Verification items for the finished model (mm, model axes). Face numbers are marked on the shaded views. A direction names the side the tool comes from. Give positions to 0.01 mm unless a question says otherwise; leave off trailing zeros. Write each loop counter-clockwise with the first axis right and the second up, starting at its lowest first coordinate (ties: lowest second). Pieces come first, ordered by that corner, then holes. Notation, with made-up numbers: (83.25, 39) -> (100.25, 39) arc R16 cw to (100.25, 63) -> close; hole circle Ø9 at (-25, 58). An arc over 180 degrees is marked (long way). Write item = value, one per line.
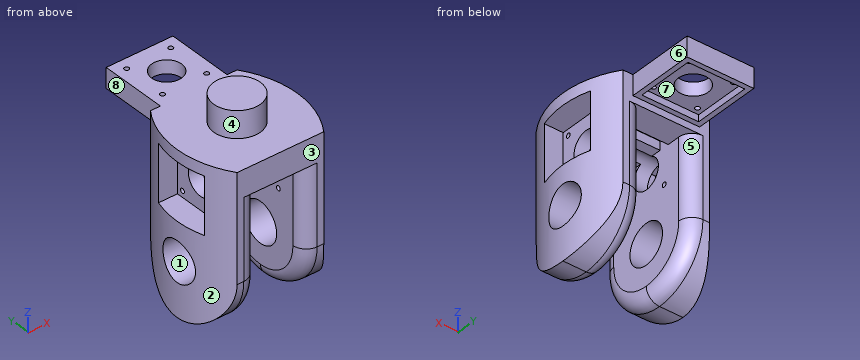
from build123d import *

# Parameters (mm, degrees)
BOSS_EXTRUDE1_DEPTH     = 100
BOSS_EXTRUDE1_2_DEPTH   = 100
BOSS_EXTRUDE2_DEPTH     = 20
SKETCH3_R               = 15
SKETCH3_R_2             = 11.25
SKETCH3_R_3             = 1.75
CUT_EXTRUDE1_DEPTH      = 46
CUT_EXTRUDE1_DEPTH_BACK = 46
SKETCH4_W               = 42.5
SKETCH4_H               = 42.5
CUT_EXTRUDE2_DEPTH      = 17.5
SKETCH5_W               = 42.5
SKETCH5_H               = 42.5
CUT_EXTRUDE4_DEPTH      = 17.5
SKETCH6_W               = 50
SKETCH6_H               = 15
BOSS_EXTRUDE3_DEPTH     = 50
SKETCH7_R               = 11.25
SKETCH7_R_2             = 1.75
CUT_EXTRUDE5_DEPTH      = 106.0000001
CUT_EXTRUDE5_DEPTH_BACK = 16.0000001
SKETCH8_W               = 42.5
SKETCH8_H               = 42.5
CUT_EXTRUDE6_DEPTH      = 5
SKETCH9_R               = 17.5
BOSS_EXTRUDE4_DEPTH     = 20
FILLET1_R               = 10
CUT_EXTRUDE7_DEPTH      = 17.5
CUT_EXTRUDE7_DEPTH_BACK = 17.5


with BuildPart() as part:
    # Sketch1 → Boss-Extrude1 (new body)
    with BuildSketch(Plane.XY):
        with BuildLine():
            Line((-17.5, -40), (-17.5, 40))
            Line((-17.5, 40), (-32.5, 40))
            ThreePointArc((-32.5, 40), (-45, 0), (-32.5, -40))
            Line((-32.5, -40), (-17.5, -40))
        make_face()
    extrude(amount=BOSS_EXTRUDE1_DEPTH)



with BuildPart() as body_2:
    # Sketch1 → Boss-Extrude1 2 (new body)
    with BuildSketch(Plane.XY):
        with BuildLine():
            Line((17.5, -40), (17.5, 40))
            Line((17.5, 40), (32.5, 40))
            ThreePointArc((32.5, 40), (45, 0), (32.5, -40))
            Line((32.5, -40), (17.5, -40))
        make_face()
    extrude(amount=BOSS_EXTRUDE1_2_DEPTH)


with BuildPart() as part_1:
    add(part.part)

    add(body_2.part)  # Boss-Extrude2 merges body 2
    # Sketch2 → Boss-Extrude2 (add)
    with BuildSketch(Plane.XY.offset(100)):
        with BuildLine():
            Line((-32.5, 40), (32.5, 40))
            ThreePointArc((32.5, 40), (45, 0), (32.5, -40))
            Line((32.5, -40), (-32.5, -40))
            ThreePointArc((-32.5, -40), (-45, 0), (-32.5, 40))
        make_face()
    extrude(amount=BOSS_EXTRUDE2_DEPTH)

    # Sketch3 → Cut-Extrude1 (cut, two sides)
    with BuildSketch(Plane(origin=(0, 0, 0), x_dir=(0, 0, -1), z_dir=(1, 0, 0))) as cut_extrude1_sk:
        with BuildLine():
            ThreePointArc((-40, 40), (-11.715728753, 28.284271247), (0, 0))
            Line((0, 0), (0, 40))
            Line((0, 40), (-40, 40))
        make_face()
        with BuildLine():
            Line((0, -40), (0, 0))
            ThreePointArc((0, 0), (-11.715728753, -28.284271247), (-40, -40))
            Line((-40, -40), (0, -40))
        make_face()
        with Locations((-40, 0)):
            Circle(SKETCH3_R)
        with Locations((-90, 0)):
            Circle(SKETCH3_R_2)
        with Locations((-73.45, -16.55)):
            Circle(SKETCH3_R_3)
        with Locations((-73.45, 16.55)):
            Circle(SKETCH3_R_3)
        with Locations((-106.55, 16.55)):
            Circle(SKETCH3_R_3)
        with Locations((-106.55, -16.55)):
            Circle(SKETCH3_R_3)
    extrude(amount=CUT_EXTRUDE1_DEPTH, mode=Mode.SUBTRACT)
    extrude(cut_extrude1_sk.sketch, amount=-CUT_EXTRUDE1_DEPTH_BACK, mode=Mode.SUBTRACT)

    # Sketch4 → Cut-Extrude2 (cut)
    with BuildSketch(Plane(origin=(45, 0, 0), x_dir=(0, 0, -1), z_dir=(1, 0, 0))):
        with Locations((-90, 0)):
            Rectangle(SKETCH4_W, SKETCH4_H)
    extrude(amount=-CUT_EXTRUDE2_DEPTH, mode=Mode.SUBTRACT)

    # Sketch5 → Cut-Extrude4 (cut)
    with BuildSketch(Plane(origin=(-45, 0, 0), x_dir=(0, 0, -1), z_dir=(1, 0, 0))):
        with Locations((-90, 0)):
            Rectangle(SKETCH5_W, SKETCH5_H)
    extrude(amount=CUT_EXTRUDE4_DEPTH, mode=Mode.SUBTRACT)

    # Sketch6 → Boss-Extrude3 (add)
    with BuildSketch(Plane(origin=(0, 40, 0), x_dir=(1, 0, 0), z_dir=(0, 1, 0))):
        with Locations((0, -112.5)):
            Rectangle(SKETCH6_W, SKETCH6_H)
    extrude(amount=BOSS_EXTRUDE3_DEPTH)

    # Sketch7 → Cut-Extrude5 (cut, two sides)
    with BuildSketch(Plane(origin=(0, 0, 105), x_dir=(-1, 0, 0), z_dir=(0, 0, -1))) as cut_extrude5_sk:
        with Locations((0, 65)):
            Circle(SKETCH7_R)
        with Locations((16.55, 81.55)):
            Circle(SKETCH7_R_2)
        with Locations((-16.55, 81.55)):
            Circle(SKETCH7_R_2)
        with Locations((-16.55, 48.45)):
            Circle(SKETCH7_R_2)
        with Locations((16.55, 48.45)):
            Circle(SKETCH7_R_2)
    extrude(amount=CUT_EXTRUDE5_DEPTH, mode=Mode.SUBTRACT)
    extrude(cut_extrude5_sk.sketch, amount=-CUT_EXTRUDE5_DEPTH_BACK, mode=Mode.SUBTRACT)

    # Sketch8 → Cut-Extrude6 (cut)
    with BuildSketch(Plane(origin=(0, 0, 105), x_dir=(-1, 0, 0), z_dir=(0, 0, -1))):
        with Locations((0, 65)):
            Rectangle(SKETCH8_W, SKETCH8_H)
    extrude(amount=-CUT_EXTRUDE6_DEPTH, mode=Mode.SUBTRACT)

    # Sketch9 → Boss-Extrude4 (add)
    with BuildSketch(Plane.XY.offset(120)):
        Circle(SKETCH9_R)
    extrude(amount=BOSS_EXTRUDE4_DEPTH)

    # Fillet1
    fillet1_edges = [part_1.edges().sort_by_distance(p)[0] for p in [
        (17.5, 40, 70),
        (17.5, -40, 70),
        (-17.5, 0, 0),
        (17.5, 0, 0),
        (-17.5, 40, 70),
        (-17.5, -40, 70),
    ]]
    fillet(fillet1_edges, radius=FILLET1_R)

    # Sketch10 → Cut-Extrude7 (cut, two sides)
    with BuildSketch(Plane(origin=(0, 0, 0), x_dir=(0, 0, -1), z_dir=(1, 0, 0))) as cut_extrude7_sk:
        with BuildLine():
            Line((-106.55, 20.3), (-92.703309556, 20.3))
            Line((-92.703309556, 20.3), (-92.703309556, 12.8))
            Line((-92.703309556, 12.8), (-106.55, 12.8))
            ThreePointArc((-106.55, 12.8), (-110.3, 16.55), (-106.55, 20.3))
        make_face()
        with BuildLine():
            Line((-106.55, -12.8), (-92.703309556, -12.8))
            Line((-92.703309556, -12.8), (-92.703309556, -20.3))
            Line((-92.703309556, -20.3), (-106.55, -20.3))
            ThreePointArc((-106.55, -20.3), (-110.3, -16.55), (-106.55, -12.8))
        make_face()
    extrude(amount=CUT_EXTRUDE7_DEPTH, mode=Mode.SUBTRACT)
    extrude(cut_extrude7_sk.sketch, amount=-CUT_EXTRUDE7_DEPTH_BACK, mode=Mode.SUBTRACT)


solid = part_1.part
Item 1: Mould release check, pull along Y, two halves, no side actions. Record for the marked faces 1, 2 and 3: +Y half, -Y half, draft (parallel to the pull), parting line (faces both ways), or undercut.
Response values:
face_1 = undercut
face_2 = parting line
face_3 = -Y half
Item 2: Sectioned sample at A-A on y = 81.55. Record the cut outline in (x, z).
Response values:
outline = (-25, 105) -> (-21.25, 105) -> (-21.25, 110) -> (-18.3, 110) -> (-18.3, 120) -> (-25, 120) -> close; (-14.8, 110) -> (14.8, 110) -> (14.8, 120) -> (-14.8, 120) -> close; (18.3, 110) -> (21.25, 110) -> (21.25, 105) -> (25, 105) -> (25, 120) -> (18.3, 120) -> close
Item 3: Material ranges on line 1 (Y direction, x = 30, z = 76.5); line 2 (Z direction, x = -22, y = -2.5); line 3 (X direction, y = 16.5, z = 109.5), recorded low to high.
Response values:
line_1 = -40 to -21.25, 21.25 to 40
line_2 = 1.73 to 25.21, 54.79 to 79.03, 100.97 to 120
line_3 = -27.5 to -17.5, 17.5 to 27.5
Item 4: Set-up check for the marked faces 4, 5, 6, 7 and 8: record each of +Z, -Z, +X, -X, +Y, -Y from which the full face is reachable in a straight line by a thin tool's end or side.
Response values:
face_4 = +Z
face_5 = -Z, +Y
face_6 = +Z, -Z, +X, +Y
face_7 = -Z
face_8 = +Z, -Z, -X, +Y
Item 5: Sectioned sample at C-C on x = 0. Record the cut outline in (y, z), then the cut area to 3 significant figures.
Response values:
outline = (-40, 100) -> (-20.3, 100) -> (-20.3, 106.55) arc R3.75 cw to (-12.8, 106.55) -> (-12.8, 100) -> (-5.15, 100) arc R11.25 cw to (5.15, 100) -> (12.8, 100) -> (12.8, 106.55) arc R3.75 cw to (20.3, 106.55) -> (20.3, 100) -> (40, 100) -> (40, 105) -> (43.75, 105) -> (43.75, 110) -> (53.75, 110) -> (53.75, 120) -> (17.5, 120) -> (17.5, 140) -> (-17.5, 140) -> (-17.5, 120) -> (-40, 120) -> close; (76.25, 110) -> (86.25, 110) -> (86.25, 105) -> (90, 105) -> (90, 120) -> (76.25, 120) -> close
area = 2,460 mm^2
Item 6: Sectioned sample at B-B on z = 90. Record the cut outline in (x, y), then the cut area to 3 significant figures.
Response values:
outline = (-41.71, -21.25) arc R70.25 ccw to (-32.5, -40) -> (-27.5, -40) arc R10 ccw to (-17.5, -30) -> (-17.5, -11.25) -> (-27.5, -11.25) -> (-27.5, -21.25) -> close; (-41.71, 21.25) -> (-27.5, 21.25) -> (-27.5, 11.25) -> (-17.5, 11.25) -> (-17.5, 30) arc R10 ccw to (-27.5, 40) -> (-32.5, 40) arc R70.25 ccw to start; (17.5, -30) arc R10 ccw to (27.5, -40) -> (32.5, -40) arc R70.25 ccw to (41.71, -21.25) -> (27.5, -21.25) -> (27.5, -11.25) -> (17.5, -11.25) -> close; (17.5, 11.25) -> (27.5, 11.25) -> (27.5, 21.25) -> (41.71, 21.25) arc R70.25 ccw to (32.5, 40) -> (27.5, 40) arc R10 ccw to (17.5, 30) -> close
area = 1,830 mm^2
Item 7: Sectioned sample at D-D on z = 62. Record the cut outline in (x, y), then the cut area to 3 significant figures.
Response values:
outline = (-32.5, -40) -> (-27.5, -40) arc R10 ccw to (-17.5, -30) -> (-17.5, 30) arc R10 ccw to (-27.5, 40) -> (-32.5, 40) arc R70.25 ccw to start; (17.5, -30) arc R10 ccw to (27.5, -40) -> (32.5, -40) arc R70.25 ccw to (32.5, 40) -> (27.5, 40) arc R10 ccw to (17.5, 30) -> close
area = 3,670 mm^2
Item 8: Go/stop test with flat-tipped pins: P1, Ø4, axis at y = 61, z = 108, coming from the +X side; P2, Ø5, axis at x = 8, z = 103, coming from the +Y side; P3, Ø2.5, axis at x = 0, y = 9, coming from the -Z side; P4, Ø12, axis at y = -18.5, z = 38.5, coming from the +X side. Record where each tip stops, or that it passes through.
Response values:
P1 = 25
P2 = 90
P3 = 100
P4 = 43.6
